```python
from build123d import *

# Parameters (mm, degrees)
EXTRUDE1_DEPTH     = 3.175
CUT_EXTRUDE1_REACH = 5.175


with BuildPart() as part:
    # Sketch1 → Extrude1 (new body)
    with BuildSketch(Plane.XY):
        Polygon((-14.605, 15.875), (-3.175, 15.875), (-3.175, 12.7), (3.175, 12.7), (3.175, 15.875), (14.605, 15.875), (14.605, 3.175), (17.78, 3.175), (17.78, -3.175), (14.605, -3.175), (14.605, -15.875), (3.175, -15.875), (-3.175, -15.875), (-14.605, -15.875), (-14.605, -3.175), (-17.78, -3.175), (-17.78, 3.175), (-14.605, 3.175), align=None)
    extrude(amount=EXTRUDE1_DEPTH)

    # Sketch2 → Cut-Extrude1 (cut, up to next)
    with BuildSketch(Plane.XY.offset(3.175), mode=Mode.PRIVATE) as cut_extrude1_sk1:
        Polygon((3.175, 2.54), (12.065, 11.43), (12.065, 2.54), align=None)
    cut_extrude1_tool1 = extrude(cut_extrude1_sk1.sketch, amount=-CUT_EXTRUDE1_REACH, mode=Mode.PRIVATE) & part.part
    add(cut_extrude1_tool1.solids().sort_by_distance((9.101667, 5.503333, 3.175))[0], mode=Mode.SUBTRACT)
    # Sketch2 → Cut-Extrude1 (cut, up to next)
    with BuildSketch(Plane.XY.offset(3.175), mode=Mode.PRIVATE) as cut_extrude1_sk2:
        Polygon((-12.065, 2.54), (-3.175, 2.54), (-12.065, 11.43), align=None)
    cut_extrude1_tool2 = extrude(cut_extrude1_sk2.sketch, amount=-CUT_EXTRUDE1_REACH, mode=Mode.PRIVATE) & part.part
    add(cut_extrude1_tool2.solids().sort_by_distance((-9.101667, 5.503333, 3.175))[0], mode=Mode.SUBTRACT)
    # Sketch2 → Cut-Extrude1 (cut, up to next)
    with BuildSketch(Plane.XY.offset(3.175), mode=Mode.PRIVATE) as cut_extrude1_sk3:
        Polygon((-3.175, -2.54), (-12.065, -11.43), (-12.065, -2.54), align=None)
    cut_extrude1_tool3 = extrude(cut_extrude1_sk3.sketch, amount=-CUT_EXTRUDE1_REACH, mode=Mode.PRIVATE) & part.part
    add(cut_extrude1_tool3.solids().sort_by_distance((-9.101667, -5.503333, 3.175))[0], mode=Mode.SUBTRACT)
    # Sketch2 → Cut-Extrude1 (cut, up to next)
    with BuildSketch(Plane.XY.offset(3.175), mode=Mode.PRIVATE) as cut_extrude1_sk4:
        Polygon((12.065, -2.54), (3.175, -2.54), (12.065, -11.43), align=None)
    cut_extrude1_tool4 = extrude(cut_extrude1_sk4.sketch, amount=-CUT_EXTRUDE1_REACH, mode=Mode.PRIVATE) & part.part
    add(cut_extrude1_tool4.solids().sort_by_distance((9.101667, -5.503333, 3.175))[0], mode=Mode.SUBTRACT)
    # Sketch2 → Cut-Extrude1 (cut, up to next)
    with BuildSketch(Plane.XY.offset(3.175), mode=Mode.PRIVATE) as cut_extrude1_sk5:
        Polygon((-7.522107489, 11.43), (7.522107489, 11.43), (0, 3.778290122), align=None)
    cut_extrude1_tool5 = extrude(cut_extrude1_sk5.sketch, amount=-CUT_EXTRUDE1_REACH, mode=Mode.PRIVATE) & part.part
    add(cut_extrude1_tool5.solids().sort_by_distance((0, 8.87943, 3.175))[0], mode=Mode.SUBTRACT)
    # Sketch2 → Cut-Extrude1 (cut, up to next)
    with BuildSketch(Plane.XY.offset(3.175), mode=Mode.PRIVATE) as cut_extrude1_sk6:
        Polygon((0, -3.778290122), (7.522107489, -11.43), (-7.522107489, -11.43), align=None)
    cut_extrude1_tool6 = extrude(cut_extrude1_sk6.sketch, amount=-CUT_EXTRUDE1_REACH, mode=Mode.PRIVATE) & part.part
    add(cut_extrude1_tool6.solids().sort_by_distance((0, -8.87943, 3.175))[0], mode=Mode.SUBTRACT)


solid = part.part
```
Can you work these out from the model? Positions are in its coordinate system, mm. A direction names the side the tool comes from. Give positions to 0.01 mm unless a question says otherwise; leave off trailing zeros. Order: outer loops, then holes, each group sorted by start corner. A loop starts at its lowest first (then second) coordinate and runs counter-clockwise, first axis right, second up. Notation, with made-up numbers: (27.5, 1.25) - (62.5, 1.25) arc R21 cw to (62.5, 27.25) - close; hole circle Ø3 at (61, -4). An arc over 180 degrees is marked (long way). Use a Markdown table: item, result. Add a question column.
Q1. On a 3-axis mill with a long thin cutter (end or side, diameter ignored), from which of +Z, -Z, +X, -X, +Y, -Y can I reach the whole of each face in a straight line? I mean faces 5 (the flat face through (3.175, 14, 2)), 6 (the flat face through (-14.605, -10, 2)), 7 (the flat face through (-14.605, 9, 2)), 8 (the flat face through (16, 3.175, 2)). Say none if no direction works.
Q2. If we section it at D-D on x = -10: Write out the boundary of the cut face in (y, z) (3 decimals), plus the area to 3 significant figures.
Q3. If we section it at A-A on y = -4.5: Write out the boundary of the cut face in (x, z) (3 decimals).
Q4. Please list where these lines run through material, in increasing order: line 1 along Y through (x, z) = (10.5, 2.15) (3 decimals); line 2 along Y through (x, z) = (-2.5, 0.95) (3 decimals); line 3 along X through (y, z) = (-4.5, 2.35) (3 decimals).
Q5. If we section it at C-C on z = 2.1: Count the separate pieces of the cut face and the enclosed holes in it, plus the area to 3 significant figures.
Q6. If we mould it in two halves opening along X, with no side actions, what happens to faces 1 (the flat face through (-7.558, -6.923, 1.61)), 2 (the flat face through (-17.78, 0, 2)), 3 (the flat face through (3.71, -7.55, 1.61)), 4 (the flat face through (0, -15.875, 2))? For each: released by +X, released by -X, zero draft, split by the parting line, or undercut.
Q7. If we section it at B-B on x = -5: Write out the boundary of the cut face in (y, z) (3 decimals).
Q8. I'm going to push flat-ended pins straight in: pin 1 (1 mm diameter, centred on y = 9, z = 1.5, fed in from +X) (3 decimals); pin 2 (1.6 mm diameter, centred on x = 16, z = 1, fed in from -Y) (3 decimals); pin 3 (1.6 mm diameter, centred on x = -17, z = 2, fed in from +Y) (3 decimals). Where does each tip first touch, or does it pass through?
Answers follow:
| question | item | result |
|---|---|---|
| 1 | face 5 | +Z, -Z, +Y |
| 1 | face 6 | +Z, -Z, -X, -Y |
| 1 | face 7 | +Z, -Z, -X, +Y |
| 1 | face 8 | +Z, -Z, +X, +Y |
| 2 | outline | (-15.875, 0) - (-9.365, 0) - (-9.365, 3.175) - (-15.875, 3.175) - close; (-2.54, 0) - (2.54, 0) - (2.54, 3.175) - (-2.54, 3.175) - close; (9.365, 0) - (15.875, 0) - (15.875, 3.175) - (9.365, 3.175) - close |
| 2 | area | 57.5 mm^2 |
| 3 | outline | (-14.605, 0) - (-12.065, 0) - (-12.065, 3.175) - (-14.605, 3.175) - close; (-5.135, 0) - (-0.709, 0) - (-0.709, 3.175) - (-5.135, 3.175) - close; (0.709, 0) - (5.135, 0) - (5.135, 3.175) - (0.709, 3.175) - close; (12.065, 0) - (14.605, 0) - (14.605, 3.175) - (12.065, 3.175) - close |
| 4 | line 1 | y = -15.875 to -9.865, -2.54 to 2.54, 9.865 to 15.875 |
| 4 | line 2 | y = -15.875 to -11.43, -6.321 to 6.321, 11.43 to 12.7 |
| 4 | line 3 | x = -14.605 to -12.065, -5.135 to -0.709, 0.709 to 5.135, 12.065 to 14.605 |
| 5 | separate pieces | 1 |
| 5 | enclosed holes | 6 |
| 5 | area | 674 mm^2 |
| 6 | face 1 | undercut |
| 6 | face 2 | released by -X |
| 6 | face 3 | undercut |
| 6 | face 4 | zero draft |
| 7 | outline | (-15.875, 0) - (-11.43, 0) - (-11.43, 3.175) - (-15.875, 3.175) - close; (-8.864, 0) - (-4.365, 0) - (-4.365, 3.175) - (-8.864, 3.175) - close; (-2.54, 0) - (2.54, 0) - (2.54, 3.175) - (-2.54, 3.175) - close; (4.365, 0) - (8.864, 0) - (8.864, 3.175) - (4.365, 3.175) - close; (11.43, 0) - (15.875, 0) - (15.875, 3.175) - (11.43, 3.175) - close |
| 8 | pin 1 | stops at x = 14.605 |
| 8 | pin 2 | stops at y = -3.175 |
| 8 | pin 3 | stops at y = 3.175 |
